Design review of the part built by this model. Coordinates are the model's own, in mm. A direction names the side the tool comes from. Coordinates: 2 decimals unless noted, no trailing zeros. Write each loop counter-clockwise with the first axis right and the second up, starting at its lowest first coordinate (ties: lowest second). Pieces come first, ordered by that corner, then holes. Notation, with made-up numbers: (37, 85) - (62, 85) arc R24 cw to (62, 123) - close; hole circle Ø4 at (39, 17.5). An arc over 180 degrees is marked (long way). Answer as a JSON object with one key per item and string values.
```python
from build123d import *

# Parameters (mm, degrees)
SKETCH1_W           = 20
SKETCH1_H           = 20
BOSS_EXTRUDE1_DEPTH = 200
SKETCH3_R           = 5
CUT_EXTRUDE1_DEPTH  = 57
SKETCH4_W           = 20
SKETCH4_H           = 4
BOSS_EXTRUDE2_DEPTH = 20
SKETCH5_R           = 5
CUT_EXTRUDE2_DEPTH  = 49


with BuildPart() as part:
    # Sketch1 → Boss-Extrude1 (new body)
    with BuildSketch(Plane.XY):
        Rectangle(SKETCH1_W, SKETCH1_H)
    extrude(amount=BOSS_EXTRUDE1_DEPTH)

    # Sketch3 → Cut-Extrude1 (cut)
    with BuildSketch(Plane.ZY.offset(10)):
        with Locations(Location((15, 0, 0), (0, 0, 270))):
            Circle(SKETCH3_R)
        with Locations(Location((185, 0, 0), (0, 0, 270))):
            Circle(SKETCH3_R)
    extrude(amount=-CUT_EXTRUDE1_DEPTH, mode=Mode.SUBTRACT)

    # Sketch4 → Boss-Extrude2 (add)
    with BuildSketch(Plane(origin=(0, 10, 0), x_dir=(1, 0, 0), z_dir=(0, 1, 0))):
        with Locations((0, -114.625901795)):
            Rectangle(SKETCH4_W, SKETCH4_H)
        with Locations((0, -90.625901795)):
            Rectangle(SKETCH4_W, SKETCH4_H)
    extrude(amount=BOSS_EXTRUDE2_DEPTH)

    # Sketch5 → Cut-Extrude2 (cut)
    with BuildSketch(Plane(origin=(0, 0, 88.625901795), x_dir=(-1, 0, 0), z_dir=(0, 0, -1))):
        with Locations((0, 23)):
            Circle(SKETCH5_R)
    extrude(amount=-CUT_EXTRUDE2_DEPTH, mode=Mode.SUBTRACT)


solid = part.part
```
(1) Take a section at A-A, the plane x = 0. Write out the cut boundary in (y, z), and give its area (3 significant figures).
Solved:
{"outline": "(-10, 0) - (10, 0) - (10, 88.63) - (18, 88.63) - (18, 92.63) - (10, 92.63) - (10, 112.63) - (18, 112.63) - (18, 116.63) - (10, 116.63) - (10, 200) - (-10, 200) - close; (28, 88.63) - (30, 88.63) - (30, 92.63) - (28, 92.63) - close; (28, 112.63) - (30, 112.63) - (30, 116.63) - (28, 116.63) - close; hole circle Ø10 at (0, 15); hole circle Ø10 at (0, 185)", "area": "3,920 mm^2"}
(2) Take a section at D-D, the plane x = 7.75. Write out the cut boundary in (y, z), and give its area (3 significant figures).
Solved:
{"outline": "(-10, 0) - (10, 0) - (10, 88.63) - (30, 88.63) - (30, 92.63) - (10, 92.63) - (10, 112.63) - (30, 112.63) - (30, 116.63) - (10, 116.63) - (10, 200) - (-10, 200) - close; hole circle Ø10 at (0, 15); hole circle Ø10 at (0, 185)", "area": "4,000 mm^2"}
(3) Take a section at C-C, the plane z = 15. Write out the cut boundary in (x, y), and give its area (3 significant figures).
Solved:
{"outline": "(-10, -10) - (10, -10) - (10, -5) - (-10, -5) - close; (-10, 5) - (10, 5) - (10, 10) - (-10, 10) - close", "area": "200 mm^2"}
(4) For pin 1 (8 mm diameter, centred on x = 3, z = 72, fed in from +Y); pin 2 (6 mm diameter, centred on x = 1, y = 16, fed in from -Z); pin 3 (6 mm diameter, centred on x = -2.5, y = 21, fed in from +Z), all flat-tipped, find the tip position at first contact; note any pin that passes through.
Solved:
{"pin 1": "stops at y = 10", "pin 2": "stops at z = 88.63", "pin 3": "stops at z = 116.63"}
(5) Take a section at B-B, the plane y = 0. Write out the cut boundary in (x, z), and give its area (3 significant figures).
Solved:
{"outline": "(-10, 0) - (10, 0) - (10, 10) - (-10, 10) - close; (-10, 20) - (10, 20) - (10, 180) - (-10, 180) - close; (-10, 190) - (10, 190) - (10, 200) - (-10, 200) - close", "area": "3,600 mm^2"}
(6) Tool access review of faces 1 (the face through (-0.1, 17.6, 116.626)), 2 (the face through (0, 10, 102)), 3 (the face through (-0.1, 17.6, 88.626)): name each direction out of +Z, -Z, +X, -X, +Y, -Y from which nothing blocks a thin tool from reaching the whole face with its end or side.
Solved:
{"face 1": "+Z, +X, -X, +Y", "face 2": "+X, -X, +Y", "face 3": "-Z, +X, -X, +Y"}
(7) To check wall thickness, follow line 1 (Z direction, x = 2.5, y = 0); line 2 (Z direction, x = 5, y = 26.5); line 3 (Y direction, x = 0, z = 90). State the ranges of each line that lie inside material, in increasing order. Write a range as from..to.
Solved:
{"line 1": "z = 0..10, 20..180, 190..200", "line 2": "z = 88.63..92.63, 112.63..116.63", "line 3": "y = -10..18, 28..30"}
(8) The part is to be moulded in two halves that separate along Y. For faces 4 (the face through (0, 30, 115)), 5 (the face through (-0.14, 0.651, 189.957)), 6 (the face through (0, -10, 99)), 7 (the face through (-0.1, 17.6, 112.626)), say which applies: pulls with the +Y half, pulls with the -Y half, needs draft (parallel to the pull), parting line crosses it, or undercut.
Solved:
{"face 4": "pulls with the +Y half", "face 5": "undercut", "face 6": "pulls with the -Y half", "face 7": "needs draft"}
